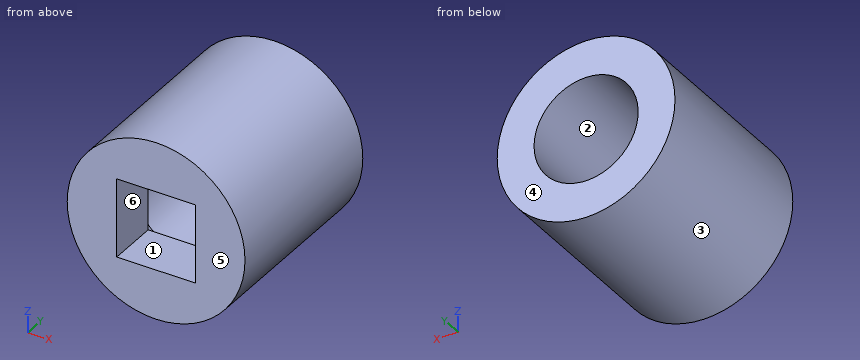
```python
from build123d import *

# Parameters (mm, degrees)
SKETCH1_R           = 7
BOSS_EXTRUDE3_DEPTH = 15
SKETCH4_R           = 4.1
CUT_EXTRUDE1_DEPTH  = 11
SKETCH5_W           = 6.2
SKETCH5_H           = 6.2
CUT_EXTRUDE2_DEPTH  = 4


with BuildPart() as part:
    # Sketch1 → Boss-Extrude3 (new body)
    with BuildSketch(Plane(origin=(0, 0, 0), x_dir=(1, 0, 0), z_dir=(0, 1, 0))):
        with Locations(Location((0, 0, 0), (0, 0, 270))):  # turned: the seam where the file's is
            Circle(SKETCH1_R)
    extrude(amount=BOSS_EXTRUDE3_DEPTH)

    # Sketch4 → Cut-Extrude1 (cut)
    with BuildSketch(Plane(origin=(0, 15, 0), x_dir=(1, 0, 0), z_dir=(0, 1, 0))):
        with Locations(Location((0, 0, 0), (0, 0, 270))):  # turned: the seam where the file's is
            Circle(SKETCH4_R)
    extrude(amount=-CUT_EXTRUDE1_DEPTH, mode=Mode.SUBTRACT)

    # Sketch5 → Cut-Extrude2 (cut)
    with BuildSketch(Plane.XZ):
        Rectangle(SKETCH5_W, SKETCH5_H)
    extrude(amount=-CUT_EXTRUDE2_DEPTH, mode=Mode.SUBTRACT)


solid = part.part
```
Source: CAD feature listing. Evaluate the final solid. Frame: model axes, mm. Face numbers are marked on the shaded views. A direction names the side the tool comes from. Round coordinates to 2 decimals unless told otherwise and drop trailing zeros. Loops run counter-clockwise (first coordinate to the right, second up) from the corner with the lowest first, then second, coordinate; pieces in that order, holes last.
1. Access query for the marked faces 1, 2 and 3. Directions: +Z, -Z, +X, -X, +Y, -Y. A direction counts if a zero-diameter tool reaches every point of the face in a straight line with its end or side. Return the directions, or none.
2. Ray query, L1, parallel to X at y = 11, z = 0; L2, parallel to X at y = 7.5, z = 2; L3, parallel to Z at x = 0.75, y = 3.75. Return the intervals inside material, ascending.
3. Section query A-A on x = 0. Output: boundary loops of the cut face in (y, z).
4. Section query C-C on y = 2.5. Output: boundary loops of the cut face in (x, z).
5. Contact query for flat-ended pins moving along their axis: pin 1 (6 mm diameter, centred on x = 0.5, z = 0.5, fed in from +Y); pin 2 (6 mm diameter, centred on x = 4.5, y = 5.5, fed in from -Z); pin 3 (3 mm diameter, centred on x = -2, y = 8, fed in from -Z). Output: stop coordinate, or through.
6. Section query D-D on z = 3.5. Output: boundary loops of the cut face in (x, y).
7. Mould query, pull axis Y, two halves, no side actions, for the marked faces 4, 5 and 6. Classes: released by +Y, released by -Y, zero draft, split by the parting line, or undercut.
8. Section query B-B on z = 0. Output: boundary loops of the cut face in (x, y).
Answers below:
1. face 1: -Y
1. face 2: +Y
1. face 3: +Y, -Y
2. L1: x = -7 to -4.1, 4.1 to 7
2. L2: x = -6.71 to -3.58, 3.58 to 6.71
2. L3: z = -6.96 to -3.1, 3.1 to 6.96
3. outline: (0, -7) - (15, -7) - (15, -4.1) - (4, -4.1) - (4, -3.1) - (0, -3.1) - close; (0, 3.1) - (4, 3.1) - (4, 4.1) - (15, 4.1) - (15, 7) - (0, 7) - close
4. outline: circle Ø14 at (0, 0); hole (-3.1, -3.1) - (3.1, -3.1) - (3.1, 3.1) - (-3.1, 3.1) - close
5. pin 1: stops at y = 4
5. pin 2: stops at z = -6.84
5. pin 3: stops at z = -6.98
6. outline: (-6.06, 0) - (6.06, 0) - (6.06, 15) - (2.14, 15) - (2.14, 4) - (-2.14, 4) - (-2.14, 15) - (-6.06, 15) - close
7. face 4: released by +Y
7. face 5: released by -Y
7. face 6: zero draft
8. outline: (-7, 0) - (-3.1, 0) - (-3.1, 4) - (-4.1, 4) - (-4.1, 15) - (-7, 15) - close; (3.1, 0) - (7, 0) - (7, 15) - (4.1, 15) - (4.1, 4) - (3.1, 4) - close
